Check sheet for the modelled part. Datum: model origin and axes. Units: mm. A direction names the side the tool comes from. Coordinates: 2 decimals unless noted, no trailing zeros. Loops run counter-clockwise (first coordinate to the right, second up) from the corner with the lowest first, then second, coordinate; pieces in that order, holes last. Notation, with made-up numbers: (62.5, 30.5) - (107.5, 30.5) arc R20 cw to (107.5, 46.5) - close; hole circle Ø7 at (-1, 44). An arc over 180 degrees is marked (long way). Use a Markdown table: item, result. Add a question column.
1) Thickness scan on line 1 (X direction, y = 31.45, z = 15.5); line 2 (X direction, y = 33.9, z = 0); line 3 (Y direction, x = 18.5, z = 5). Record the ranges inside material, lowest first.
2) Sectioned sample at A-A, the plane x = 0. Enter the section's corners in (y, z).
3) Draft check along X on faces 1 (the flat face through (-5, 34, -14.4)), 2 (the flat face through (21.15, 17, 0)), 3 (the cylindrical face through (-15.43, 32.03, 14)). Enter one of: pulls with the +X half, pulls with the -X half, needs draft (parallel to the pull), parting line crosses it, or undercut.
4) Sectioned sample at C-C, the plane y = 45. Enter the section's corners in (x, z), then the cut area to 3 significant figures.
5) Go/stop test with flat-tipped pins: P1, Ø3.5, axis at x = -15, z = -16, coming from the +Y side; P2, Ø3, axis at x = 9, z = -14.5, coming from the -Y side; P3, Ø6, axis at y = 49.5, z = 1.5, coming from the +X side; P4, Ø1.5, axis at x = 15.5, z = 15.5, coming from the +Y side. Record where each tip stops, or that it passes through.
6) Tool access check on faces 4 (the flat face through (-21.15, 17, 0)), 5 (the cylindrical face through (-15.43, 32.03, -17)). Record the directions out of +Z, -Z, +X, -X, +Y, -Y that give a thin tool (end or side, any length) a straight path to the whole face; none if there is none.
7) Sectioned sample at B-B, the plane z = -1.5. Enter the section's corners in (x, y).
8) Sectioned sample at D-D, the plane x = 9.5. Enter the section's corners in (y, z), then the cut area to 3 significant figures.
from build123d import *

# Parameters (mm, degrees)
SKETCH1_W            = 42.3
SKETCH1_H            = 42.3
BODY_DEPTH           = 34
SKETCH2_R            = 1.5
MOUNTING_HOLES_DEPTH = 4
SKETCH3_R            = 11
CENTER_THING_DEPTH   = 2
SKETCH4_R            = 2.5
SHAFT_DEPTH          = 22
LARGE_DIVOT_START    = -0.2
SKETCH5_R            = 15
SKETCH5_R_2          = 11
LARGE_DIVOT_DEPTH    = 0.2


with BuildPart() as part:
    # Sketch1 → body (new body)
    with BuildSketch(Plane(origin=(0, 0, 0), x_dir=(1, 0, 0), z_dir=(0, 1, 0))):
        Rectangle(SKETCH1_W, SKETCH1_H)
    extrude(amount=BODY_DEPTH)

    # Sketch2 → mounting-holes (cut)
    with BuildSketch(Plane(origin=(0, 34, 0), x_dir=(1, 0, 0), z_dir=(0, 1, 0))):
        with Locations(Location((-15.5, 15.5, 0), (0, 0, 270))):
            Circle(SKETCH2_R)
        with Locations(Location((15.5, 15.5, 0), (0, 0, 270))):
            Circle(SKETCH2_R)
        with Locations(Location((15.5, -15.5, 0), (0, 0, 270))):
            Circle(SKETCH2_R)
        with Locations(Location((-15.5, -15.5, 0), (0, 0, 270))):
            Circle(SKETCH2_R)
    extrude(amount=-MOUNTING_HOLES_DEPTH, mode=Mode.SUBTRACT)

    # Sketch3 → center-thing (add)
    with BuildSketch(Plane(origin=(0, 34, 0), x_dir=(1, 0, 0), z_dir=(0, 1, 0))):
        with Locations(Location((0, 0, 0), (0, 0, 270))):
            Circle(SKETCH3_R)
    extrude(amount=CENTER_THING_DEPTH)

    # Sketch4 → shaft (add)
    with BuildSketch(Plane(origin=(0, 36, 0), x_dir=(1, 0, 0), z_dir=(0, 1, 0))):
        with Locations(Location((0, 0, 0), (0, 0, 270))):
            Circle(SKETCH4_R)
    extrude(amount=SHAFT_DEPTH)

    # Sketch5 → large-divot (cut)
    with BuildSketch(Plane(origin=(0, 34, 0), x_dir=(1, 0, 0), z_dir=(0, 1, 0)).offset(LARGE_DIVOT_START)):
        with Locations(Location((0, 0, 0), (0, 0, 270))):
            Circle(SKETCH5_R)
        with Locations(Location((0, 0, 0), (0, 0, 270))):
            Circle(SKETCH5_R_2, mode=Mode.SUBTRACT)
    extrude(amount=LARGE_DIVOT_DEPTH, mode=Mode.SUBTRACT)


solid = part.part
Solved:
| question | item | result |
|---|---|---|
| 1 | line 1 | x = -21.15 to -17, -14 to 14, 17 to 21.15 |
| 1 | line 2 | x = -21.15 to -15, -11 to 11, 15 to 21.15 |
| 1 | line 3 | y = 0 to 34 |
| 2 | outline | (0, -21.15) - (34, -21.15) - (34, -15) - (33.8, -15) - (33.8, -11) - (36, -11) - (36, -2.5) - (58, -2.5) - (58, 2.5) - (36, 2.5) - (36, 11) - (33.8, 11) - (33.8, 15) - (34, 15) - (34, 21.15) - (0, 21.15) - close |
| 3 | face 1 | needs draft |
| 3 | face 2 | pulls with the +X half |
| 3 | face 3 | undercut |
| 4 | outline | circle Ø5 at (0, 0) |
| 4 | area | 19.6 mm2 |
| 5 | P1 | stops at y = 34 |
| 5 | P2 | stops at y = 0 |
| 5 | P3 | stops at x = 2.5 |
| 5 | P4 | stops at y = 30 |
| 6 | face 4 | +Z, -Z, -X, +Y, -Y |
| 6 | face 5 | +Y |
| 7 | outline | (-21.15, 0) - (21.15, 0) - (21.15, 34) - (14.92, 34) - (14.92, 33.8) - (10.9, 33.8) - (10.9, 36) - (2, 36) - (2, 58) - (-2, 58) - (-2, 36) - (-10.9, 36) - (-10.9, 33.8) - (-14.92, 33.8) - (-14.92, 34) - (-21.15, 34) - close |
| 8 | outline | (0, -21.15) - (34, -21.15) - (34, -11.61) - (33.8, -11.61) - (33.8, -5.55) - (36, -5.55) - (36, 5.55) - (33.8, 5.55) - (33.8, 11.61) - (34, 11.61) - (34, 21.15) - (0, 21.15) - close |
| 8 | area | 1,460 mm2 |
